For this review, take the finished solid that the model builds, in its own axes (mm). Face numbers are marked on the shaded views. A direction names the side the tool comes from. Coordinates: 2 decimals unless noted, no trailing zeros. Loops run counter-clockwise (first coordinate to the right, second up) from the corner with the lowest first, then second, coordinate; pieces in that order, holes last. Notation, with made-up numbers: (43.5, -3) - (66.5, -3) arc R13 cw to (66.5, 4) - close; hole circle Ø8 at (23.5, -20). An arc over 180 degrees is marked (long way). One line per item, written item: value. Start each with the question number.
1. Insertion check: pin 1 (1.7 mm diameter, centred on x = 10.5, z = 1, fed in from +Y); pin 2 (2.5 mm diameter, centred on y = 3.5, z = 3, fed in from -X); pin 3 (2.5 mm diameter, centred on x = 9, z = 1, fed in from -Y); pin 4 (2.5 mm diameter, centred on x = 3.25, y = 3.25, fed in from +Z). Each pin has a flat end and moves straight along its axis. Give the tip position at first contact, or say it passes through.
2. To check wall thickness, follow line 1 (Z direction, x = 9.25, y = 3.25); line 2 (X direction, y = 3.25, z = 0.7); line 3 (Z direction, x = 0.75, y = 3). State the ranges of each line that lie inside material, in increasing order. Write a range as from..to.
3. Take a section at B-B, the plane y = 3.75. State the section outline as (x, z) points, and give its area (3 significant figures).
4. Take a section at C-C, the plane z = 3.1. State the section outline as (x, y) points, and give its area (3 significant figures).
5. The part is to be moulded in two halves that separate along Y. For the marked faces 4, 5, 6 and 7, say which applies: released by +Y, released by -Y, zero draft, split by the parting line, or undercut.
6. Take a section at D-D, the plane x = 3.75. State the section outline as (y, z) points.
7. For the marked faces 1, 2 and 3, list the 3-axis set-ups (+Z, -Z, +X, -X, +Y, -Y) from which the entire face can be reached by the end or side of a thin tool; tool diameter is ignored.
```python
from build123d import *

# Parameters (mm, degrees)
F0_R     = 1.6
F1_DEPTH = 0.95
F2_W     = 4.5
F2_H     = 4.2
F3_DEPTH = 3.25
F4_R     = 2.09999
F5_R     = 1.15
F6_DEPTH = 25


# Not quite as in the source:
# - a fillet or chamfer is up to 0.001 mm smaller than in the source, because OpenCascade refuses the exact size


with BuildPart() as f1:
    # F0 (on Top) → F1 (new body)
    with BuildSketch(Plane.XY):
        with BuildLine():
            Line((7.7320977576, 1.15), (12.7, 1.15))
            Line((12.7, 1.15), (12.7, 5.35))
            Line((12.7, 5.35), (8.2, 5.35))
            Line((8.2, 5.35), (7.7320977576, 5.35))
            ThreePointArc((7.7320977576, 5.35), (7.2069912058, 5.3927015871), (6.6956833513, 5.5196842405))
            Line((6.6956833513, 5.5196842405), (4.2864144063, 6.3303157595))
            ThreePointArc((4.2864144063, 6.3303157595), (3.7751065518, 6.4572984129), (3.25, 6.5))
            ThreePointArc((3.25, 6.5), (0.9519029611, 5.5480970389), (0, 3.25))
            ThreePointArc((0, 3.25), (0.9519029611, 0.9519029611), (3.25, 0))
            ThreePointArc((3.25, 0), (3.7751065518, 0.0427015871), (4.2864144063, 0.1696842405))
            Line((4.2864144063, 0.1696842405), (6.6956833513, 0.9803157595))
            ThreePointArc((6.6956833513, 0.9803157595), (7.2069912058, 1.1072984129), (7.7320977576, 1.15))
        make_face()
        with Locations((3.25, 3.25)):
            Circle(F0_R, mode=Mode.SUBTRACT)
    extrude(amount=F1_DEPTH)

    # F2 (on face) → F3 (join)
    with BuildSketch(Plane.XY.offset(0.95)):
        with Locations((10.45, 3.25)):
            Rectangle(F2_W, F2_H)
    extrude(amount=F3_DEPTH)

    # F4 (radius 2.1 in the source; OpenCascade refuses exactly that, so slightly less here)
    f4_edges = [f1.edges().sort_by_distance(p)[0] for p in [
        (10.45, 5.35, 4.2),
        (10.45, 1.15, 4.2),
    ]]
    fillet(f4_edges, radius=F4_R)

    # F5 (on face) → F6 (cut)
    with BuildSketch(Plane.YZ.offset(12.7)):
        with Locations((3.25, 2.1)):
            Circle(F5_R)
    extrude(amount=-F6_DEPTH, mode=Mode.SUBTRACT)


solid = f1.part
```
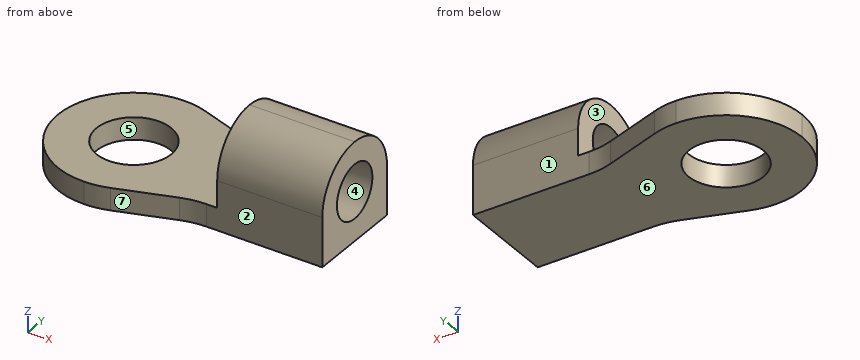
Solutions:
1. pin 1: y = 5.35
1. pin 2: x = 8.2
1. pin 3: y = 1.15
1. pin 4: through
2. line 1: 0..0.95, 3.25..4.2
2. line 2: 0..1.65, 4.85..12.7
2. line 3: 0..0.95
3. outline: (0.04, 0) - (1.73, 0) - (1.73, 0.95) - (0.04, 0.95) - close; (4.77, 0) - (12.7, 0) - (12.7, 1.06) - (8.2, 1.06) - (8.2, 0.95) - (4.77, 0.95) - close; (8.2, 3.14) - (12.7, 3.14) - (12.7, 4.14) - (8.2, 4.14) - close
3. area: 14.2 mm2
4. outline: (8.2, 1.4) - (12.7, 1.4) - (12.7, 2.68) - (8.2, 2.68) - close; (8.2, 3.82) - (12.7, 3.82) - (12.7, 5.1) - (8.2, 5.1) - close
4. area: 11.5 mm2
5. face 4: undercut
5. face 5: undercut
5. face 6: zero draft
5. face 7: released by -Y
6. outline: (0.04, 0) - (1.73, 0) - (1.73, 0.95) - (0.04, 0.95) - close; (4.77, 0) - (6.46, 0) - (6.46, 0.95) - (4.77, 0.95) - close
7. face 1: +Z, -Z, +X, +Y
7. face 2: +Z, -Z, +X, -Y
7. face 3: +Z, -X, +Y, -Y
